The model under review builds one solid part; all positions refer to its coordinate system, in mm. Face numbers are marked on the shaded views. Round coordinates to 2 decimals unless told otherwise and drop trailing zeros. Order: outer loops, then holes, each group sorted by start corner. A loop starts at its lowest first (then second) coordinate and runs counter-clockwise, first axis right, second up.
1) Consider section D-D (y = 0). Give the boundary of the cut face in (x, z), then the cut area to 3 significant figures.
2) Consider section A-A (y = -2). Give the boundary of the cut face in (x, z), then the cut area to 3 significant figures.
3) Clearance check with a flat-ended pin moving along its axis: P1, Ø5, axis at x = 14.5, y = -1.5, coming from the -Z side. State where the tip first meets the part, or that it passes through.
4) Consider section C-C (z = 2.15). Give the boundary of the cut face in (x, y).
5) To check wall thickness, follow L1, parallel to X at y = -0.5, z = 2.25; L2, parallel to X at y = -1.25, z = 0.9; L3, parallel to Y at x = 0, z = 2.25. State the ranges of each line that lie inside material, in increasing order.
6) Consider section B-B (x = -15). Give the boundary of the cut face in (y, z).
7) Mouldability with a two-part tool opening along X and no side actions: class the marked faces 1, 2 and 3 as pulls with the +X half, pulls with the -X half, needs draft (parallel to the pull), parting line crosses it, or undercut.
from build123d import *

# Parameters (mm, degrees)
SKETCH_1_W      = 40
SKETCH_1_H      = 10
SKETCH_1_R      = 2.5
EXTRUDE_1_DEPTH = 3


with BuildPart() as part:
    # 草圖1 → 填料-伸長1 (new body)
    with BuildSketch(Plane.XY):
        Rectangle(SKETCH_1_W, SKETCH_1_H)
        with Locations((-15, 0)):
            Circle(SKETCH_1_R, mode=Mode.SUBTRACT)
        with Locations((15, 0)):
            Circle(SKETCH_1_R, mode=Mode.SUBTRACT)
        Circle(SKETCH_1_R, mode=Mode.SUBTRACT)
    extrude(amount=EXTRUDE_1_DEPTH)


solid = part.part
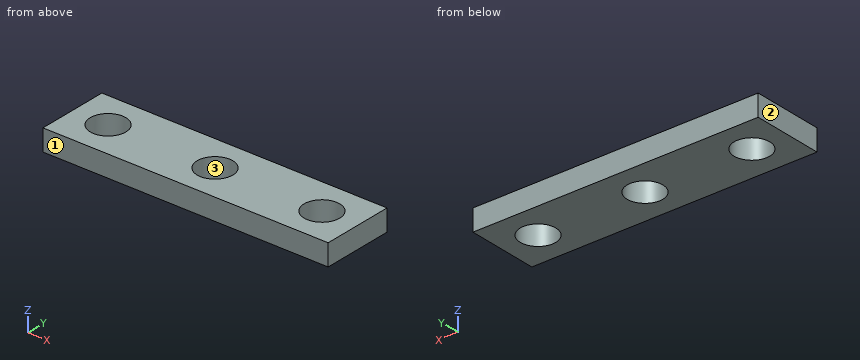
Answer below:
1. outline: (-20, 0) - (-17.5, 0) - (-17.5, 3) - (-20, 3) - close; (-12.5, 0) - (-2.5, 0) - (-2.5, 3) - (-12.5, 3) - close; (2.5, 0) - (12.5, 0) - (12.5, 3) - (2.5, 3) - close; (17.5, 0) - (20, 0) - (20, 3) - (17.5, 3) - close
1. area: 75.0 mm2
2. outline: (-20, 0) - (-16.5, 0) - (-16.5, 3) - (-20, 3) - close; (-13.5, 0) - (-1.5, 0) - (-1.5, 3) - (-13.5, 3) - close; (1.5, 0) - (13.5, 0) - (13.5, 3) - (1.5, 3) - close; (16.5, 0) - (20, 0) - (20, 3) - (16.5, 3) - close
2. area: 93.0 mm2
3. P1: stops at z = 0
4. outline: (-20, -5) - (20, -5) - (20, 5) - (-20, 5) - close; hole circle Ø5 at (-15, 0); hole circle Ø5 at (0, 0); hole circle Ø5 at (15, 0)
5. L1: x = -20 to -17.45, -12.55 to -2.45, 2.45 to 12.55, 17.45 to 20
5. L2: x = -20 to -17.17, -12.83 to -2.17, 2.17 to 12.83, 17.17 to 20
5. L3: y = -5 to -2.5, 2.5 to 5
6. outline: (-5, 0) - (-2.5, 0) - (-2.5, 3) - (-5, 3) - close; (2.5, 0) - (5, 0) - (5, 3) - (2.5, 3) - close
7. face 1: needs draft
7. face 2: pulls with the -X half
7. face 3: undercut
